Here's the drawing with two shaded views (mm, measured from the low corner). I have some questions. A direction names the side the tool comes from. Give positions to 0.01 mm unless a question says otherwise; leave off trailing zeros. Loops run counter-clockwise (first coordinate to the right, second up) from the corner with the lowest first, then second, coordinate; pieces in that order, holes last. Notation, with made-up numbers: (-29.5, 7.25) - (-24.5, 7.25) arc R23 cw to (-24.5, 39.25) - close; hole circle Ø9 at (30.5, 86). An arc over 180 degrees is marked (long way). Answer as a JSON object with one key per item and string values. Group by question number.
Item 1: Will this pin go through, and if not, where does the flat tip stop? pin 1 (1 mm diameter, centred on y = 3.5, z = 4.5, fed in from +X).
Item 2: Suppose I cut it at B-B on y = 3.5. Write out the boundary of the cut face in (x, z), and give its area (3 significant figures).
Item 3: Thinking about a two-plate mould opening in Y: for the marked faces 3 and 4, which applies, pulls with the +Y half, pulls with the -Y half, needs draft (parallel to the pull), parting line crosses it, or undercut?
Item 4: Which directions (+Z, -Z, +X, -X, +Y, -Y) give clear straight access to the entire face, cutting with the end or side of a thin tool? Please do the marked faces 1 and 2.
Item 5: Suppose I cut it at D-D on x = 1.5. Write out the boundary of the cut face in (y, z).
Item 6: Please list where these lines run through material, in increasing order: L1, parallel to X at y = 6.5, z = 2; L2, parallel to X at y = 3.75, z = 3; L3, parallel to Z at x = 14.25, y = 5.75.
Item 7: Suppose I cut it at A-A on z = 3.5. Write out the boundary of the cut face in (x, y), and give its area (3 significant figures).
Item 8: Suppose I cut it at C-C on x = 10.75. Write out the boundary of the cut face in (y, z).
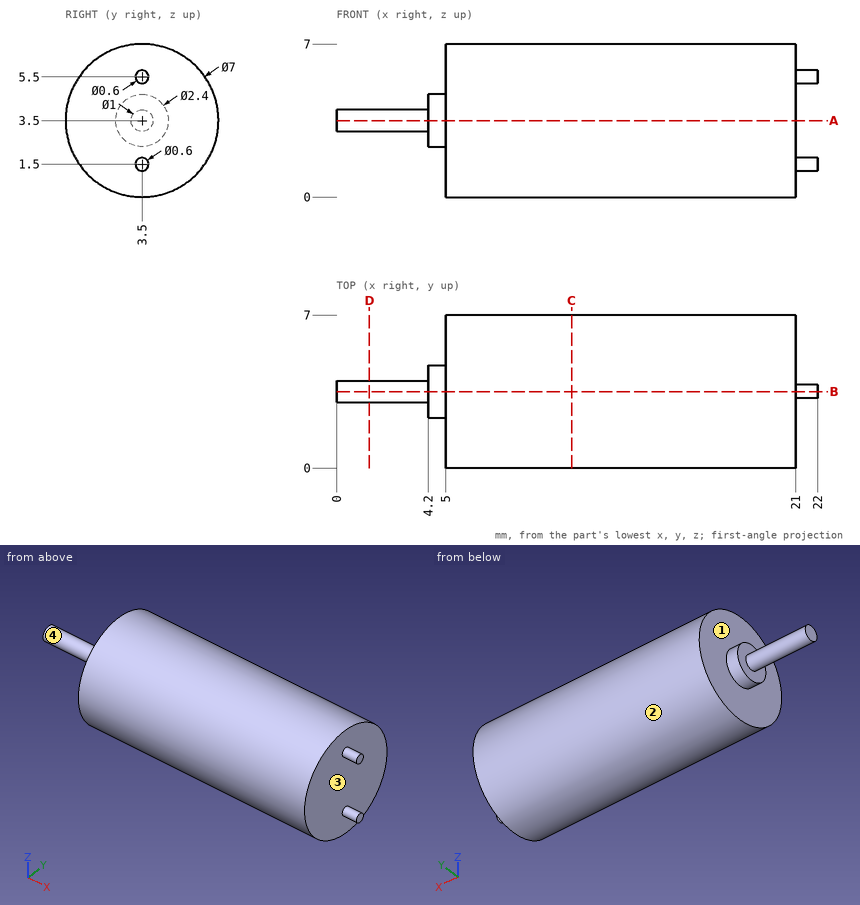
Worked out:
{
 "1": {"pin 1": "stops at x = 21"},
 "2": {"outline": "(0, 3) - (4.2, 3) - (4.2, 2.3) - (5, 2.3) - (5, 0) - (21, 0) - (21, 1.2) - (22, 1.2) - (22, 1.8) - (21, 1.8) - (21, 5.2) - (22, 5.2) - (22, 5.8) - (21, 5.8) - (21, 7) - (5, 7) - (5, 4.7) - (4.2, 4.7) - (4.2, 4) - (0, 4) - close", "area": "119 mm2"},
 "3": {"face 3": "needs draft", "face 4": "parting line crosses it"},
 "4": {"face 1": "-X", "face 2": "+X, -X"},
 "5": {"outline": "circle Ø1 at (3.5, 3.5)"},
 "6": {"L1": "x = 5 to 21", "L2": "x = 4.2 to 21", "L3": "z = 0.82 to 6.18"},
 "7": {"outline": "(0, 3) - (4.2, 3) - (4.2, 2.3) - (5, 2.3) - (5, 0) - (21, 0) - (21, 7) - (5, 7) - (5, 4.7) - (4.2, 4.7) - (4.2, 4) - (0, 4) - close", "area": "118 mm2"},
 "8": {"outline": "circle Ø7 at (3.5, 3.5)"}
}
